Verification items for this drawing (mm, ordinates from the low corner). A direction names the side the tool comes from. Round coordinates to 2 decimals unless told otherwise and drop trailing zeros. Order: outer loops, then holes, each group sorted by start corner. A loop starts at its lowest first (then second) coordinate and runs counter-clockwise, first axis right, second up. Notation, with made-up numbers: (-20.5, -37.75) -> (-3.5, -37.75) arc R8 ccw to (-3.5, -31.75) -> close; hole circle Ø7 at (-35.75, 87.5). An arc over 180 degrees is marked (long way). Return JSON: item names as keys, results as strings. Group by question number.
Item 1: Sectioned sample at B-B on z = 5.5. Record the cut outline in (x, y).
Item 2: Scan lines: probe 1 along X at (y, z) = (29.5, 28); probe 2 along Z at (x, y) = (3.75, 34); probe 3 along Y at (x, z) = (16.25, 19.5). Record each from-to range of solid material in increasing order. Write a range as from..to.
Item 3: Access from +Z, -Z, +X, -X, +Y, -Y to the whole of each face (thin tool, end or side, straight path). Record for the marked faces 1 and 2.
Item 4: Sectioned sample at C-C on y = 30. Record the cut outline in (x, z), plus the area to 3 significant figures.
Item 5: Depth check by flat-ended pin: pin 1 Ø5 at (x, y) = (5.5, 9) entering from +Z; pin 2 Ø6 at (y, z) = (27.5, 16) entering from -X; pin 3 Ø12 at (x, z) = (7.5, 14.5) entering from +Y. Enter the tip coordinate at first touch or a pass-through.
Item 6: Sectioned sample at A-A on x = 15.5. Record the cut outline in (y, z).
Item 7: Sectioned sample at D-D on y = 8. Record the cut outline in (x, z).
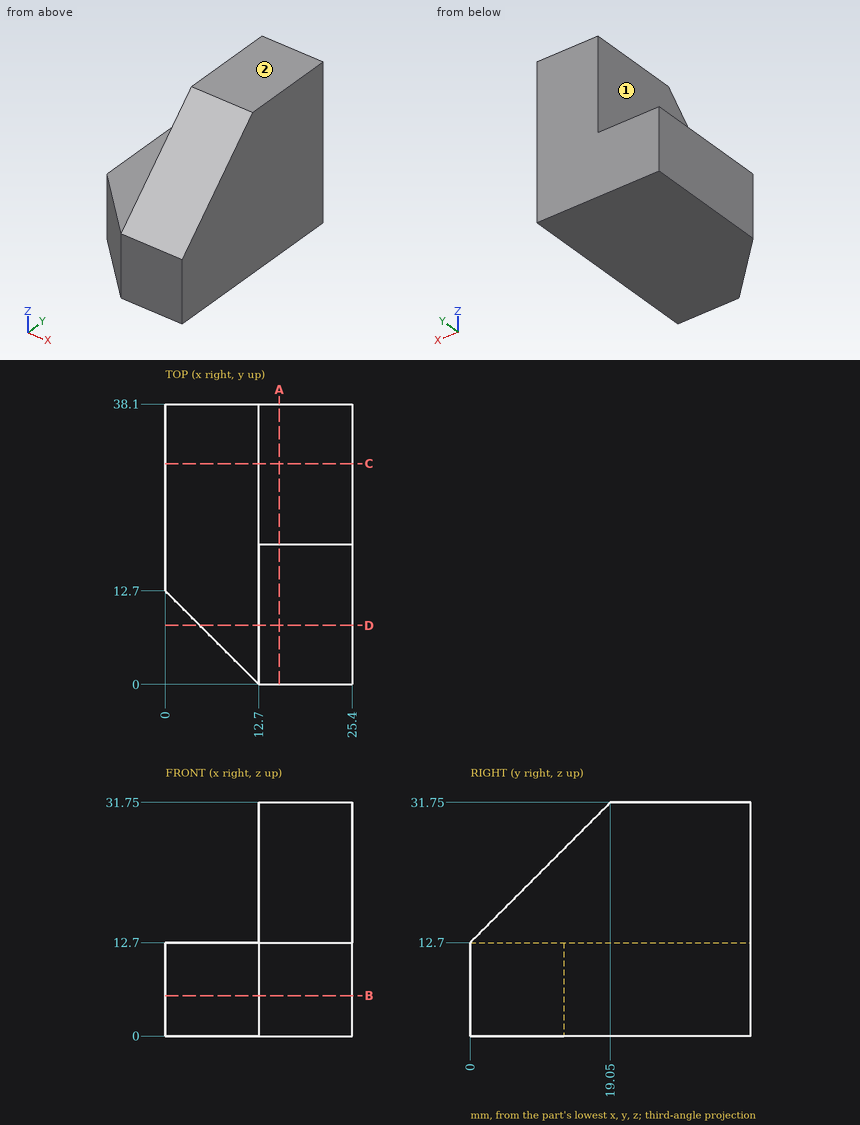
Recorded:
{
 "1": {"outline": "(0, 12.7) -> (12.7, 0) -> (25.4, 0) -> (25.4, 38.1) -> (0, 38.1) -> close"},
 "2": {"probe 1": "12.7..25.4", "probe 2": "0..12.7", "probe 3": "6.8..38.1"},
 "3": {"face 1": "+Z, -X, +Y, -Y", "face 2": "+Z, +X, -X, +Y, -Y"},
 "4": {"outline": "(0, 0) -> (25.4, 0) -> (25.4, 31.75) -> (12.7, 31.75) -> (12.7, 12.7) -> (0, 12.7) -> close", "area": "565 mm²"},
 "5": {"pin 1": "z = 12.7", "pin 2": "x = 12.7", "pin 3": "y = 38.1"},
 "6": {"outline": "(0, 0) -> (38.1, 0) -> (38.1, 31.75) -> (19.05, 31.75) -> (0, 12.7) -> close"},
 "7": {"outline": "(4.7, 0) -> (25.4, 0) -> (25.4, 20.7) -> (12.7, 20.7) -> (12.7, 12.7) -> (4.7, 12.7) -> close"}
}
